Could you check a few things on this model? Use its own coordinates, in mm. A direction names the side the tool comes from. Round coordinates to 2 decimals unless told otherwise and drop trailing zeros. Loops run counter-clockwise (first coordinate to the right, second up) from the corner with the lowest first, then second, coordinate; pieces in that order, holes last. Notation, with made-up numbers: (-8, 70) - (-1, 70) arc R33 cw to (-1, 107) - close; hole circle Ø7 at (0, 41.25). An arc over 180 degrees is marked (long way). Put each result on its own line as item: value. Start each with the question number.
from build123d import *

# Parameters (mm, degrees)
F0_W     = 40
F0_H     = 40
F1_DEPTH = 10
F2_W     = 40
F2_H     = 40
F2_W_2   = 25
F2_H_2   = 2.5
F2_W_3   = 5.5
F2_H_3   = 13
F2_R     = 5
F3_DEPTH = 11
F4_DEPTH = 5
F5_SIZE  = 1


with BuildPart() as f1:
    # F0 (on Top) → F1 (new body)
    with BuildSketch(Plane.XY):
        Rectangle(F0_W, F0_H)
    extrude(amount=F1_DEPTH)

    # F2 (on face) → F3 (join)
    with BuildSketch(Plane.XY.offset(10)):
        Rectangle(F2_W, F2_H)
        with Locations((0, -13.75)):
            Rectangle(F2_W_2, F2_H_2, mode=Mode.SUBTRACT)
        with Locations((-12.25, 0)):
            Rectangle(F2_W_3, F2_H_3, mode=Mode.SUBTRACT)
        Circle(F2_R, mode=Mode.SUBTRACT)
        with Locations((12.25, 0)):
            Rectangle(F2_W_3, F2_H_3, mode=Mode.SUBTRACT)
        with Locations((0, 13.75)):
            Rectangle(F2_W_2, F2_H_2, mode=Mode.SUBTRACT)
    extrude(amount=F3_DEPTH)

    # F4 (cut): a face of the model
    f4_faces = [f1.faces().sort_by_distance(p)[0] for p in [
        (0, 0, 10),
    ]]
    extrude(f4_faces, amount=-F4_DEPTH, mode=Mode.SUBTRACT)

    # F5
    f5_edges = [f1.edges().sort_by_distance(p)[0] for p in [
        (0, -20, 21),
        (20, 0, 21),
        (0, 20, 21),
        (-20, 0, 21),
        (0, -12.5, 21),
        (12.5, -13.75, 21),
        (0, -15, 21),
        (-12.5, -13.75, 21),
        (-12.25, 6.5, 21),
        (-9.5, 0, 21),
        (-12.25, -6.5, 21),
        (-15, 0, 21),
        (-5, 0, 21),
        (12.25, 6.5, 21),
        (15, 0, 21),
        (12.25, -6.5, 21),
        (9.5, 0, 21),
        (0, 15, 21),
        (12.5, 13.75, 21),
        (0, 12.5, 21),
        (-12.5, 13.75, 21),
    ]]
    chamfer(f5_edges, length=F5_SIZE)


solid = f1.part
Item 1: Suppose I cut it at C-C, the plane y = 0. List the corners of the cut face in (x, z) for me, then the cut area to 3 significant figures.
Item 2: Suppose I cut it at B-B, the plane z = 16.5. List the corners of the cut face in (x, y) for me.
Item 3: On a 3-axis mill with a long thin cutter (end or side, diameter ignored), from which of +Z, -Z, +X, -X, +Y, -Y can I reach the whole of each face in a straight line? I mean faces 1 (the face through (0, 0, 0)), 2 (the face through (9, -0.1, 20.5)). Say none if no direction works.
Item 4: Suppose I cut it at A-A, the plane x = 0. List the corners of the cut face in (y, z) for me.
Item 5: I need wall thicknesses on line 1 (Y direction, x = 0, z = 13.5); line 2 (Y direction, x = 12, z = 14.5); line 3 (Y direction, x = 5.5, z = 10.5). Which ranges of each line are inside material? Lowest first, please. Write a range as from..to.
Item 6: Will these pins go through, and if not, where does the flat tip stop? P1, Ø0.8, axis at x = 2.5, y = -13.5, coming from the +Z side; P2, Ø4.5, axis at x = 11.5, y = 2, coming from the +Z side.
Item 7: Thinking about a two-plate mould opening in Y: for faces 3 (the face through (-0.3, 19.5, 20.5)), 4 (the face through (19.5, -0.3, 20.5)), 5 (the face through (13, -13.8, 20.5)), which applies, released by +Y, released by -Y, zero draft, split by the parting line, or undercut?
Numbers:
1. outline: (-20, 0) - (20, 0) - (20, 20) - (19, 21) - (16, 21) - (15, 20) - (15, 10) - (9.5, 10) - (9.5, 20) - (8.5, 21) - (6, 21) - (5, 20) - (5, 5) - (-5, 5) - (-5, 20) - (-6, 21) - (-8.5, 21) - (-9.5, 20) - (-9.5, 10) - (-15, 10) - (-15, 20) - (-16, 21) - (-19, 21) - (-20, 20) - close
1. area: 555 mm^2
2. outline: (-20, -20) - (20, -20) - (20, 20) - (-20, 20) - close; hole (-15, -6.5) - (-9.5, -6.5) - (-9.5, 6.5) - (-15, 6.5) - close; hole (-12.5, -15) - (12.5, -15) - (12.5, -12.5) - (-12.5, -12.5) - close; hole (-12.5, 12.5) - (12.5, 12.5) - (12.5, 15) - (-12.5, 15) - close; hole circle Ø10 at (0, 0); hole (9.5, -6.5) - (15, -6.5) - (15, 6.5) - (9.5, 6.5) - close
3. face 1: -Z, +X, -X, +Y, -Y
3. face 2: +Z
4. outline: (-20, 0) - (20, 0) - (20, 20) - (19, 21) - (16, 21) - (15, 20) - (15, 10) - (12.5, 10) - (12.5, 20) - (11.5, 21) - (6, 21) - (5, 20) - (5, 5) - (-5, 5) - (-5, 20) - (-6, 21) - (-11.5, 21) - (-12.5, 20) - (-12.5, 10) - (-15, 10) - (-15, 20) - (-16, 21) - (-19, 21) - (-20, 20) - close
5. line 1: -20..-15, -12.5..-5, 5..12.5, 15..20
5. line 2: -20..-15, -12.5..-6.5, 6.5..12.5, 15..20
5. line 3: -20..-15, -12.5..12.5, 15..20
6. P1: z = 10
6. P2: z = 20.25
7. face 3: released by +Y
7. face 4: zero draft
7. face 5: undercut
